Build history of the part. All positions in model axes, mm. A direction names the side the tool comes from. Give positions to 0.01 mm unless a question says otherwise; leave off trailing zeros. Write each loop counter-clockwise with the first axis right and the second up, starting at its lowest first coordinate (ties: lowest second). Pieces come first, ordered by that corner, then holes. Notation, with made-up numbers: M 84,12.25 L 100,12.25 A6 ccw 100,18.25 Z; hole C 70.5,-33.5 d1. An arc over 180 degrees is marked long. One line per item, written item: value. Start each with the question number.
from build123d import *

# Parameters (mm, degrees)
F0_R     = 6.5
F0_R_2   = 5.5
F1_DEPTH = 2.5
F0_R_3   = 3
F0_R_4   = 2
F2_DEPTH = 2


with BuildPart() as f1:
    # F0 (on Top) → F1 (new body, symmetric)
    with BuildSketch(Plane.XY):
        Circle(F0_R)
        Circle(F0_R_2, mode=Mode.SUBTRACT)
    extrude(amount=F1_DEPTH, both=True)



with BuildPart() as f1b:
    # F0 (on Top) → F1, piece 2 (new body, symmetric)
    with BuildSketch(Plane.XY):
        Circle(F0_R_3)
        Circle(F0_R_4, mode=Mode.SUBTRACT)
    extrude(amount=F1_DEPTH, both=True)


with BuildPart() as f1_1:
    add(f1.part)

    add(f1b.part)  # F2 merges F1b
    # F0 (on Top) → F2 (join, symmetric)
    with BuildSketch(Plane.XY):
        Circle(F0_R_2)
        Circle(F0_R_3, mode=Mode.SUBTRACT)
    extrude(amount=F2_DEPTH, both=True)


solid = f1_1.part
1) Drop flat-ended pins along their axis: P1, Ø1, axis at x = -2, z = -2, coming from the -Y side; P2, Ø3, axis at y = 1, z = -1.5, coming from the -X side; P3, Ø1, axis at x = -1.5, y = 3.5, coming from the +Z side. Give the stop position or say it passes through.
2) Band-saw the part on A-A (x = 0). List the corners of the cut face in (y, z), then the cut area to 3 significant figures.
3) Mould opens along X. For faces 1 (the face through (1, -2, -2.5)), 2 (the face through (2.4, -2.4, -2)), 3 (the face through (-5.158, -3.955, 0.035)), 4 (the face through (-1.19, -5.37, 2.25)) say: released by +X, released by -X, zero draft, split by the parting line, or undercut.
4) Tool access for faces 5 (the face through (-1.19, -5.37, -2.25)), 6 (the face through (2.4, -2.4, 2)), 7 (the face through (-5, 3, -2.5)): list every direction of +Z, -Z, +X, -X, +Y, -Y with a clear straight run to the whole face (end or side of a thin tool).
5) Probe line 1 along Y through (x, z) = (0, 2.15); line 2 along Z through (x, y) = (-3.75, -2); line 3 along X through (y, z) = (-0.5, 1.45). List the from-to ranges inside material, lowest first. Write a range as from..to.
6) Band-saw the part on D-D (x = -5). List the corners of the cut face in (y, z), then the cut area to 3 significant figures.
7) Band-saw the part on C-C (z = 0.15). List the corners of the cut face in (x, y).
Model answer:
1. P1: stops at y = -6.32
1. P2: stops at x = -6.5
1. P3: stops at z = 2
2. outline: M -6.5,-2.5 L -5.5,-2.5 L -5.5,-2 L -3,-2 L -3,-2.5 L -2,-2.5 L -2,2.5 L -3,2.5 L -3,2 L -5.5,2 L -5.5,2.5 L -6.5,2.5 Z; M 2,-2.5 L 3,-2.5 L 3,-2 L 5.5,-2 L 5.5,-2.5 L 6.5,-2.5 L 6.5,2.5 L 5.5,2.5 L 5.5,2 L 3,2 L 3,2.5 L 2,2.5 Z
2. area: 40.0 mm²
3. face 1: zero draft
3. face 2: undercut
3. face 3: split by the parting line
3. face 4: undercut
4. face 5: -Z
4. face 6: +Z
4. face 7: -Z, +X, -X, +Y, -Y
5. line 1: y = -6.5..-5.5, -3..-2, 2..3, 5.5..6.5
5. line 2: z = -2..2
5. line 3: x = -6.48..-1.94, 1.94..6.48
6. outline: M -4.15,-2.5 L -2.29,-2.5 L -2.29,-2 L 2.29,-2 L 2.29,-2.5 L 4.15,-2.5 L 4.15,2.5 L 2.29,2.5 L 2.29,2 L -2.29,2 L -2.29,2.5 L -4.15,2.5 Z
6. area: 37.0 mm²
7. outline: C 0,0 d13; hole C 0,0 d4
